Study the drawing (mm; zero at the part's minimum x, y, z) and answer. Coordinates: 2 decimals unless noted, no trailing zeros. Write each loop counter-clockwise with the first axis right and the second up, starting at its lowest first coordinate (ties: lowest second). Pieces come first, ordered by that corner, then holes. Notation, with made-up numbers: M 26,-20 L 74,-20 A21 cw 74,17 Z; hole C 14.25,52.5 d6. An arc over 180 degrees is marked long. Answer as a JSON object with one key per item and string values. Group by question number.
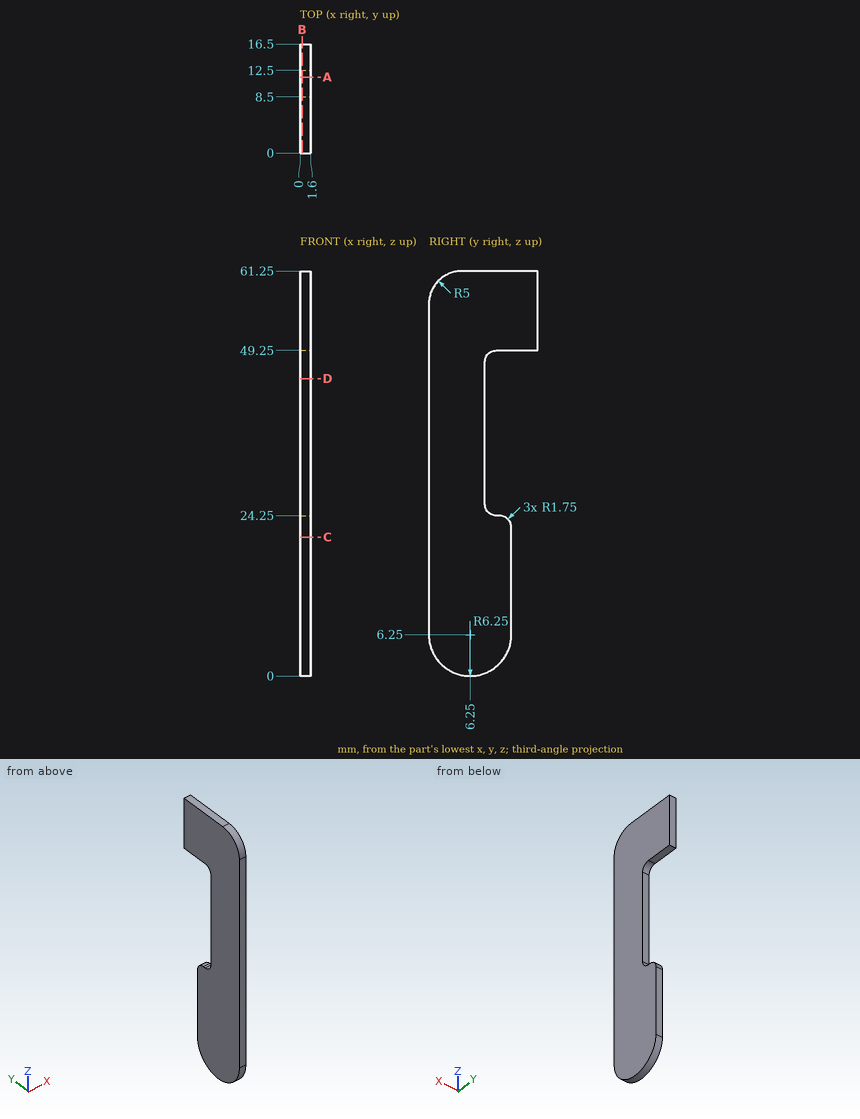
Item 1: Consider L1, parallel to Z at x = 1, y = 13.5; L2, parallel to Y at x = 0.7, z = 38; L3, parallel to Y at x = 0.5, z = 17. Determine where each line is inside the solid, lowest interval first. Write a range as from..to.
Item 2: A cutting plane is placed at A-A, the plane y = 11.5. Write down the section's boundary in (x, z), and give its area (3 significant figures).
Item 3: Flat-ended cylindrical pins translate along their axes: pin 1 Ø0.8 at (x, z) = (0.5, 12) entering from +Y; pin 2 Ø0.5 at (x, y) = (0.5, 14.5) entering from -Z; pin 3 Ø0.5 at (x, z) = (1, 33) entering from +Y. Find the tip coordinate at first contact, or state that the pin passes through.
Item 4: A cutting plane is placed at B-B, the plane x = 0.3. Write down the section's boundary in (y, z).
Item 5: A cutting plane is placed at C-C, the plane z = 21. Write down the section's boundary in (x, y).
Item 6: A cutting plane is placed at D-D, the plane z = 45. Write down the section's boundary in (x, y), and give its area (3 significant figures).
Answer:
{
 "1": {"L1": "49.25..61.25", "L2": "0..8.5", "L3": "0..12.5"},
 "2": {"outline": "M 0,2.86 L 1.6,2.86 L 1.6,24.08 L 0,24.08 Z; M 0,49.25 L 1.6,49.25 L 1.6,61.25 L 0,61.25 Z", "area": "53.2 mm2"},
 "3": {"pin 1": "y = 12.5", "pin 2": "z = 49.25", "pin 3": "y = 8.5"},
 "4": {"outline": "M 0,6.25 A6.25 ccw 12.5,6.25 L 12.5,22.5 A1.75 ccw 10.75,24.25 L 10.25,24.25 A1.75 cw 8.5,26 L 8.5,47.5 A1.75 cw 10.25,49.25 L 16.5,49.25 L 16.5,61.25 L 5,61.25 A5 ccw 0,56.25 Z"},
 "5": {"outline": "M 0,0 L 1.6,0 L 1.6,12.5 L 0,12.5 Z"},
 "6": {"outline": "M 0,0 L 1.6,0 L 1.6,8.5 L 0,8.5 Z", "area": "13.6 mm2"}
}
